Can you work these out from the model? Positions are in its coordinate system, mm. A direction names the side the tool comes from. Round coordinates to 2 decimals unless told otherwise and drop trailing zeros. Loops run counter-clockwise (first coordinate to the right, second up) from the corner with the lowest first, then second, coordinate; pieces in that order, holes last. Notation, with made-up numbers: (19.5, -15.75) -> (48.5, -15.75) arc R21 ccw to (48.5, 10.25) -> close; hole circle Ø2 at (-16.75, 68.5). An arc over 180 degrees is marked (long way). Use a Markdown table: item, result.
from build123d import *

# Parameters (mm, degrees)
SKETCH3_W           = 12.7
SKETCH3_H           = 3.175
SKETCH3_R           = 0.999998
SKETCH3_R_2         = 10.922
BOSS_EXTRUDE1_DEPTH = 3.175


with BuildPart() as part:
    # Sketch3 → Boss-Extrude1 (new body)
    with BuildSketch(Plane.XY):
        Polygon((-20.32, -15.875), (-20.32, -19.05), (20.32, -19.05), (20.32, -15.875), (25.4, -15.875), (25.4, -1.5875), (20.32, -1.5875), (20.32, 1.5875), (25.4, 1.5875), (25.4, 15.875), (20.32, 15.875), (20.32, 19.05), (-20.32, 19.05), (-20.32, 15.875), (-25.4, 15.875), (-25.4, 1.5875), (-20.32, 1.5875), (-20.32, -1.5875), (-25.4, -1.5875), (-25.4, -15.875), align=None)
        with Locations((-11.43, -12.5095)):
            Rectangle(SKETCH3_W, SKETCH3_H, mode=Mode.SUBTRACT)
        with Locations((0, -13.611800056)):
            Circle(SKETCH3_R, mode=Mode.SUBTRACT)
        with Locations((11.43, -12.5095)):
            Rectangle(SKETCH3_W, SKETCH3_H, mode=Mode.SUBTRACT)
        with Locations((0, -5.6e-08)):
            Circle(SKETCH3_R_2, mode=Mode.SUBTRACT)
        with Locations((-13.611800056, 0)):
            Circle(SKETCH3_R, mode=Mode.SUBTRACT)
        with Locations((13.611800056, 0)):
            Circle(SKETCH3_R, mode=Mode.SUBTRACT)
        with Locations((0, 13.611800056)):
            Circle(SKETCH3_R, mode=Mode.SUBTRACT)
    extrude(amount=BOSS_EXTRUDE1_DEPTH)


solid = part.part
1. I want a section at C-C (x = 8.5). Please give me the cut outline in (y, z) (3 decimals), plus the area to 3 significant figures.
Answer sheet:
| item | result |
|---|---|
| outline | (-19.05, 0) -> (-14.097, 0) -> (-14.097, 3.175) -> (-19.05, 3.175) -> close; (-10.922, 0) -> (-6.859, 0) -> (-6.859, 3.175) -> (-10.922, 3.175) -> close; (6.859, 0) -> (19.05, 0) -> (19.05, 3.175) -> (6.859, 3.175) -> close |
| area | 67.3 mm² |
2. I need wall thicknesses on line 1 (Y direction, x = 13.5, z = 2.5); line 2 (Y direction, x = 0, z = 2.35); line 3 (Y direction, x = 9, z = 1.15). Which ranges of each line are inside material? Lowest first, please.
Answer sheet:
| item | result |
|---|---|
| line 1 | y = -19.05 to -14.1, -10.92 to -0.99, 0.99 to 19.05 |
| line 2 | y = -19.05 to -14.61, -12.61 to -10.92, 10.92 to 12.61, 14.61 to 19.05 |
| line 3 | y = -19.05 to -14.1, -10.92 to -6.19, 6.19 to 19.05 |
3. I want a section at D-D (y = 8.5). Please give me the cut outline in (x, z) (3 decimals).
Answer sheet:
| item | result |
|---|---|
| outline | (-25.4, 0) -> (-6.859, 0) -> (-6.859, 3.175) -> (-25.4, 3.175) -> close; (6.859, 0) -> (25.4, 0) -> (25.4, 3.175) -> (6.859, 3.175) -> close |
4. If we mould it in two halves opening along Y, with no side actions, what happens to faces 5 (the flat face through (-23, -15.875, 2)), 6 (the flat face through (25.4, -9, 2)), 7 (the flat face through (-20.32, 0, 2))? For each: +Y half, -Y half, draft (parallel to the pull), parting line (faces both ways), or undercut.
Answer sheet:
| item | result |
|---|---|
| face 5 | -Y half |
| face 6 | draft |
| face 7 | undercut |
5. I want a section at A-A (y = 0). Please give me the cut outline in (x, z) (3 decimals).
Answer sheet:
| item | result |
|---|---|
| outline | (-20.32, 0) -> (-14.612, 0) -> (-14.612, 3.175) -> (-20.32, 3.175) -> close; (-12.612, 0) -> (-10.922, 0) -> (-10.922, 3.175) -> (-12.612, 3.175) -> close; (10.922, 0) -> (12.612, 0) -> (12.612, 3.175) -> (10.922, 3.175) -> close; (14.612, 0) -> (20.32, 0) -> (20.32, 3.175) -> (14.612, 3.175) -> close |
6. I want a section at B-B (x = 0). Please give me the cut outline in (y, z) (3 decimals), plus the area to 3 significant figures.
Answer sheet:
| item | result |
|---|---|
| outline | (-19.05, 0) -> (-14.612, 0) -> (-14.612, 3.175) -> (-19.05, 3.175) -> close; (-12.612, 0) -> (-10.922, 0) -> (-10.922, 3.175) -> (-12.612, 3.175) -> close; (10.922, 0) -> (12.612, 0) -> (12.612, 3.175) -> (10.922, 3.175) -> close; (14.612, 0) -> (19.05, 0) -> (19.05, 3.175) -> (14.612, 3.175) -> close |
| area | 38.9 mm² |
7. Will these pins go through, and if not, where does the flat tip stop? pin 1 Ø1 at (x, z) = (-23.5, 2) entering from -Y (3 decimals); pin 2 Ø1 at (x, z) = (23.5, 1) entering from +Y (3 decimals); pin 3 Ø1 at (y, z) = (-0.5, 1) entering from -X.
Answer sheet:
| item | result |
|---|---|
| pin 1 | stops at y = -15.875 |
| pin 2 | stops at y = 15.875 |
| pin 3 | stops at x = -20.32 |
8. Which directions (+Z, -Z, +X, -X, +Y, -Y) give clear straight access to the entire face, cutting with the end or side of a thin tool? Please do faces 1 (the flat face through (-23, 1.588, 2)), 2 (the flat face through (-20.32, 17, 2)), 3 (the flat face through (20.32, -17, 2)), 4 (the flat face through (-17.78, -13, 2)).
Answer sheet:
| item | result |
|---|---|
| face 1 | +Z, -Z, -X |
| face 2 | +Z, -Z, -X, +Y |
| face 3 | +Z, -Z, +X, -Y |
| face 4 | +Z, -Z |
